For this review, take the finished solid that the model builds, in its own axes (mm). Face numbers are marked on the shaded views. A direction names the side the tool comes from. Give positions to 0.01 mm unless a question says otherwise; leave off trailing zeros. Write each loop counter-clockwise with the first axis right and the second up, starting at its lowest first coordinate (ties: lowest second). Pieces come first, ordered by that corner, then holes. Notation, with made-up numbers: M 1,68.5 L 7,68.5 A29 ccw 7,91.5 Z; hole C 11.5,-29 d7. An arc over 180 degrees is marked long. Write item = value, one per line.
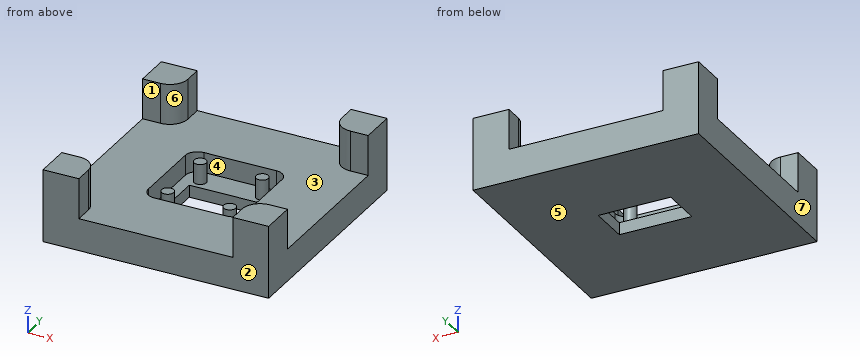
```python
from build123d import *

# Parameters (mm, degrees)
ESBO_O1_W                = 56
ESBO_O1_H                = 56
RESSALTO_EXTRUS_O1_DEPTH = 8
RESSALTO_EXTRUS_O2_DEPTH = 10
ESPELHAR2_COPY_1_DEPTH   = 10
ESBO_O3_R                = 1.5
CORTE_EXTRUS_O1_DEPTH    = 5
ESBO_O4_W                = 18
ESBO_O4_H                = 10
CORTE_EXTRUS_O2_DEPTH    = 12


with BuildPart() as part:
    # Esboço1 → Ressalto-extrusão1 (new body)
    with BuildSketch(Plane.XY):
        Rectangle(ESBO_O1_W, ESBO_O1_H)
    extrude(amount=RESSALTO_EXTRUS_O1_DEPTH)

    # Esboço2 → Ressalto-extrusão2 (add)
    with BuildSketch(Plane.XY.offset(8)):
        with BuildLine():
            Line((-19.1, 23.55), (-19.1, 28))
            Line((-19.1, 28), (-28, 28))
            Line((-28, 28), (-28, 19.1))
            Line((-28, 19.1), (-23.55, 19.1))
            ThreePointArc((-23.55, 19.1), (-20.403374824, 20.403374824), (-19.1, 23.55))
        make_face()
    ressalto_extrus_o2 = extrude(amount=RESSALTO_EXTRUS_O2_DEPTH)

    # Espelhar1: Ressalto-extrusão2 across plane
    add(ressalto_extrus_o2.mirror(Plane(origin=(0, 0, 0), x_dir=(0, 0, 1), z_dir=(1, 0, 0))))

    # Espelhar2: Ressalto-extrusão2 across plane
    add(ressalto_extrus_o2.mirror(Plane.ZX))

    # Espelhar2 copy 1 sketch → Espelhar2 copy 1 (add)
    with BuildSketch(Plane(origin=(0, 0, 8), x_dir=(-1, 0, 0), z_dir=(0, 0, 1))):
        with BuildLine():
            Line((-19.1, 23.55), (-19.1, 28))
            Line((-19.1, 28), (-28, 28))
            Line((-28, 28), (-28, 19.1))
            Line((-28, 19.1), (-23.55, 19.1))
            ThreePointArc((-23.55, 19.1), (-20.403374824, 20.403374824), (-19.1, 23.55))
        make_face()
    extrude(amount=ESPELHAR2_COPY_1_DEPTH)

    # Esboço3 → Corte-extrusão1 (cut)
    with BuildSketch(Plane.XY.offset(8)):
        with BuildLine():
            Line((9.1, -11.85), (-8.9, -11.85))
            ThreePointArc((-8.9, -11.85), (-11.021320344, -10.971320344), (-11.9, -8.85))
            Line((-11.9, -8.85), (-11.9, 8.65))
            ThreePointArc((-11.9, 8.65), (-11.021320344, 10.771320344), (-8.9, 11.65))
            Line((-8.9, 11.65), (9.1, 11.65))
            ThreePointArc((9.1, 11.65), (11.221320344, 10.771320344), (12.1, 8.65))
            Line((12.1, 8.65), (12.1, -8.85))
            ThreePointArc((12.1, -8.85), (11.221320344, -10.971320344), (9.1, -11.85))
        make_face()
        with Locations((-7.7, 7.7)):
            Circle(ESBO_O3_R, mode=Mode.SUBTRACT)
        with Locations((7.7, 7.7)):
            Circle(ESBO_O3_R, mode=Mode.SUBTRACT)
        with Locations((7.7, -7.7)):
            Circle(ESBO_O3_R, mode=Mode.SUBTRACT)
        with Locations((-7.7, -7.7)):
            Circle(ESBO_O3_R, mode=Mode.SUBTRACT)
    extrude(amount=-CORTE_EXTRUS_O1_DEPTH, mode=Mode.SUBTRACT)

    # Esboço4 → Corte-extrusão2 (cut)
    with BuildSketch(Plane.XY.offset(3)):
        Rectangle(ESBO_O4_W, ESBO_O4_H)
    extrude(amount=-CORTE_EXTRUS_O2_DEPTH, mode=Mode.SUBTRACT)


solid = part.part
```
1. Machinability: for the marked faces 1, 2 and 3, which of the approach directions +Z, -Z, +X, -X, +Y, -Y give a long, thin tool a straight path to every point of the face, cutting with its end or side? Answer none if there is none.
Responses:
face_1 = +Z, +X, -X
face_2 = +Z, -Z, +X, -X, -Y
face_3 = +Z
2. Insertion check: P1, Ø6, axis at x = -3, z = 12.5, coming from the -Y side; P2, Ø3.5, axis at x = -7, y = -8.5, coming from the +Z side. Each pin has a flat end and moves straight along its axis. Give the tip position at first contact, or say it passes through.
Responses:
P1 = through
P2 = 8
3. We need section C-C, the plane y = 7.7. Write out the cut boundary in (x, z), then the cut area to 3 significant figures.
Responses:
outline = M -28,0 L 28,0 L 28,8 L 12.1,8 L 12.1,3 L 9.2,3 L 9.2,8 L 6.2,8 L 6.2,3 L -6.2,3 L -6.2,8 L -9.2,8 L -9.2,3 L -11.9,3 L -11.9,8 L -28,8 Z
area = 358 mm2
4. For line 1 along Y through (x, z) = (-4.5, 2.25); line 2 along X through (y, z) = (-8.5, 4.75); line 3 along Y through (x, z) = (1.5, 7.25), list the stretches that pass through material, from the lowest coordinate up. Write a range as from..to.
Responses:
line_1 = -28..-5, 5..28
line_2 = -28..-11.9, -8.97..-6.43, 6.43..8.97, 12.1..28
line_3 = -28..-11.85, 11.65..28
5. We need section D-D, the plane z = 2.25. Write out the cut boundary in (x, y), then the cut area to 3 significant figures.
Responses:
outline = M -28,-28 L 28,-28 L 28,28 L -28,28 Z; hole M -9,-5 L 9,-5 L 9,5 L -9,5 Z
area = 2,960 mm2
6. We need section B-B, the plane x = -7.7. Write out the cut boundary in (y, z).
Responses:
outline = M -28,0 L -5,0 L -5,3 L -6.2,3 L -6.2,8 L -9.2,8 L -9.2,3 L -11.85,3 L -11.85,8 L -28,8 Z; M 5,0 L 28,0 L 28,8 L 11.65,8 L 11.65,3 L 9.2,3 L 9.2,8 L 6.2,8 L 6.2,3 L 5,3 Z
7. The part is to be moulded in two halves that separate along X. For the marked faces 4, 5, 6 and 7, say which applies: +X half, -X half, draft (parallel to the pull), parting line (faces both ways), or undercut.
Responses:
face_4 = undercut
face_5 = draft
face_6 = undercut
face_7 = -X half
8. We need section A-A, the plane z = 12.75. Write out the cut boundary in (x, y), then the cut area to 3 significant figures.
Responses:
outline = M -28,-28 L -19.1,-28 L -19.1,-23.55 A4.45 ccw -23.55,-19.1 L -28,-19.1 Z; M -28,19.1 L -23.55,19.1 A4.45 ccw -19.1,23.55 L -19.1,28 L -28,28 Z; M 19.1,-28 L 28,-28 L 28,-19.1 L 23.55,-19.1 A4.45 ccw 19.1,-23.55 Z; M 19.1,23.55 A4.45 ccw 23.55,19.1 L 28,19.1 L 28,28 L 19.1,28 Z
area = 300 mm2
